For this review, take the finished solid that the model builds, in its own axes (mm). A direction names the side the tool comes from. Coordinates: 2 decimals unless noted, no trailing zeros. Write each loop counter-clockwise with the first axis right and the second up, starting at its lowest first coordinate (ties: lowest second). Pieces come first, ordered by that corner, then holes.
```python
from build123d import *

# Parameters (mm, degrees)
SKETCH1_R           = 5
BOSS_EXTRUDE1_DEPTH = 76.2
SKETCH2_R           = 2.525
CUT_EXTRUDE1_DEPTH  = 6


with BuildPart() as part:
    # Sketch1 → Boss-Extrude1 (new body)
    with BuildSketch(Plane.XY):
        Circle(SKETCH1_R)
    extrude(amount=BOSS_EXTRUDE1_DEPTH)

    # Sketch2 → Cut-Extrude1 (cut)
    with BuildSketch(Plane.XY.offset(76.2)):
        Circle(SKETCH2_R)
    cut_extrude1 = extrude(amount=-CUT_EXTRUDE1_DEPTH, mode=Mode.SUBTRACT)

    # Mirror1: Cut-Extrude1 across plane
    add(cut_extrude1.mirror(Plane(origin=(0, 0, 38.1), x_dir=(1, 0, 0), z_dir=(0, 0, -1))), mode=Mode.SUBTRACT)


solid = part.part
```
Q1. Add section A-A (x = -1.75). State the section outline as (y, z) points, then the cut area to 3 significant figures.
Ans:
outline: (-4.68, 0) - (-1.82, 0) - (-1.82, 6) - (1.82, 6) - (1.82, 0) - (4.68, 0) - (4.68, 76.2) - (1.82, 76.2) - (1.82, 70.2) - (-1.82, 70.2) - (-1.82, 76.2) - (-4.68, 76.2) - close
area: 670 mm2
Q2. Add section C-C (y = 1). State the section outline as (x, z) points, then the cut area to 3 significant figures.
Ans:
outline: (-4.9, 0) - (-2.32, 0) - (-2.32, 6) - (2.32, 6) - (2.32, 0) - (4.9, 0) - (4.9, 76.2) - (2.32, 76.2) - (2.32, 70.2) - (-2.32, 70.2) - (-2.32, 76.2) - (-4.9, 76.2) - close
area: 691 mm2
Q3. Draft analysis for pull direction X (two halves, no side actions). For faces 4 (the flat face through (2, -2, 0)), 5 (the cylindrical face through (-1.08, -4.88, 37.57)), 6 (the flat face through (0, 0, 70.2)), state which applies: +X half, -X half, draft (parallel to the pull), parting line (faces both ways), or undercut.
Ans:
face 4: draft
face 5: parting line
face 6: undercut
Q4. Clearance check with flat-ended pins moving along their axes: pin 1 Ø3 at (x, y) = (0, 0) entering from -Z; pin 2 Ø3 at (y, z) = (-2, 16) entering from -X. State where each tip first meets the part, or that it passes through.
Ans:
pin 1: stops at z = 6
pin 2: stops at x = -4.97
Q5. Tool access review of faces 1 (the flat face through (2, -2, 76.2)), 2 (the cylindrical face through (2.41, 0.76, 73.24)), 3 (the cylindrical face through (2.41, 0.76, 2.96)): name each direction out of +Z, -Z, +X, -X, +Y, -Y from which nothing blocks a thin tool from reaching the whole face with its end or side.
Ans:
face 1: +Z, +X, -X, +Y, -Y
face 2: +Z
face 3: -Z
Q6. For probe 1 along Z at (x, y) = (-0.5, -0.75); probe 2 along Y at (x, z) = (0, 4.3) (3 decimals); probe 3 along X at (y, z) = (3.25, 63), list the stretches that pass through material, from the lowest coordinate up.
Ans:
probe 1: z = 6 to 70.2
probe 2: y = -5 to -2.525, 2.525 to 5
probe 3: x = -3.8 to 3.8
Q7. Add section B-B (z = 40.5). State the section outline as (x, y) points, then the cut area to 3 significant figures.
Ans:
outline: circle Ø10 at (0, 0)
area: 78.5 mm2
